Design review of the part built by this model. Coordinates are the model's own, in mm. A direction names the side the tool comes from. Coordinates: 2 decimals unless noted, no trailing zeros. Loops run counter-clockwise (first coordinate to the right, second up) from the corner with the lowest first, then second, coordinate; pieces in that order, holes last. Notation, with made-up numbers: (71.5, -27) -> (127.5, -27) arc R19 ccw to (127.5, -5) -> close; hole circle Ø8 at (43, 28.5). An arc over 180 degrees is marked (long way). One line per item, written item: value. Start each with the question number.
1. Add section A-A on x = 22. Write out the cut boundary in (y, z).
2. Draft analysis for pull direction Y (two halves, no side actions). For faces 4 (the cylindrical face through (31.1, -16.42, 11.15)), 5 (the cylindrical face through (26.06, -19.87, 12.63)), 6 (the flat face through (6, -23, 3)), state which applies: pulls with the +Y half, pulls with the -Y half, needs draft (parallel to the pull), parting line crosses it, or undercut.
3. Machinability: for faces 1 (the flat face through (31, -20.47, 12)), 2 (the cylindrical face through (-22.939, -10.265, 10.846)), 3 (the cylindrical face through (-13.08, -19.87, 12.63)), which of the approach directions +Z, -Z, +X, -X, +Y, -Y give a long, thin tool a straight path to every point of the face, cutting with its end or side? Answer none if there is none.
4. Insertion check: pin 1 (4 mm diameter, centred on x = 3.5, z = 7, fed in from -Y); pin 2 (3.5 mm diameter, centred on x = -18.5, z = 13, fed in from -Y); pin 3 (4 mm diameter, centred on x = -6, y = -21, fed in from +Z). Each pin has a flat end and moves straight along its axis. Give the tip position at first contact, or say it passes through.
5. Add section C-C on z = 16.75. Write out the cut boundary in (x, y), plus the area to 3 significant figures.
6. For probe 1 along Y at (x, z) = (-18.5, 17.75); probe 2 along X at (y, z) = (-13.25, 18.5); probe 3 along X at (y, z) = (-17, 16.75), list the stretches that pass through material, from the lowest coordinate up.
7. Add section D-D on y = -21.25. Write out the cut boundary in (x, z), plus the area to 3 significant figures.
8. Add section B-B on z = 2.25. Write out the cut boundary in (x, y).
```python
from build123d import *

# Parameters (mm, degrees)
SKETCH_1_W          = 60
SKETCH_1_H          = 20
SKETCH_1_R          = 1.5
EXTRUDE_2_DEPTH     = 3
EXTRUDE_3_DEPTH     = 19
SKETCH_3_R          = 1.8
CUT_EXTRUDE_1_DEPTH = 52.917907506
FILLET_1_R          = 2


with BuildPart() as part:
    # ｽｹｯﾁ1 → ﾎﾞｽ - 押し出し2 (new body)
    with BuildSketch(Plane.XY):
        with Locations((6.490384615, -19.663461538)):
            Rectangle(SKETCH_1_W, SKETCH_1_H)
        with Locations((30.990384615, -24.663461538)):
            Circle(SKETCH_1_R, mode=Mode.SUBTRACT)
        with Locations((-18.009615385, -24.663461538)):
            Circle(SKETCH_1_R, mode=Mode.SUBTRACT)
    extrude(amount=EXTRUDE_2_DEPTH)

    # ｽｹｯﾁ2 → ﾎﾞｽ - 押し出し3 (add)
    with BuildSketch(Plane.XY.offset(3)):
        Polygon((6.490384615, -16.663461538), (25.490384615, -16.663461538), (25.490384615, -20.47046126), (36.490384615, -20.47046126), (36.490384615, -9.663461538), (-23.509615385, -9.663461538), (-23.509615385, -20.47046126), (-12.509615385, -20.47046126), (-12.509615385, -16.663461538), align=None)
    extrude(amount=EXTRUDE_3_DEPTH)

    # ｽｹｯﾁ3 → ｶｯﾄ - 押し出し1 (cut, through all)
    with BuildSketch(Plane.XY.offset(22)):
        with Locations((31.490384615, -14.663461538)):
            Circle(SKETCH_3_R)
        with Locations((-18.509615385, -14.663461538)):
            Circle(SKETCH_3_R)
    extrude(amount=-CUT_EXTRUDE_1_DEPTH, mode=Mode.SUBTRACT)

    # ﾌｨﾚｯﾄ1
    fillet_1_edges = [part.edges().sort_by_distance(p)[0] for p in [
        (25.490384615, -20.47046126, 12.5),
        (36.490384615, -20.47046126, 12.5),
        (-23.509615385, -20.47046126, 12.5),
        (-12.509615385, -20.47046126, 12.5),
        (-23.509615385, -9.663461538, 11),
        (36.490384615, -9.663461538, 11),
        (36.490384615, -29.663461538, 1.5),
        (-23.509615385, -29.663461538, 1.5),
    ]]
    fillet(fillet_1_edges, radius=FILLET_1_R)


solid = part.part
```
Worked answers:
1. outline: (-29.66, 0) -> (-9.66, 0) -> (-9.66, 22) -> (-16.66, 22) -> (-16.66, 3) -> (-29.66, 3) -> close
2. face 4: undercut
2. face 5: pulls with the -Y half
2. face 6: needs draft
3. face 1: +Z, +X, -X, -Y
3. face 2: +Z, -Z, -X, +Y
3. face 3: +Z, -Y
4. pin 1: stops at y = -16.66
4. pin 2: stops at y = -20.47
4. pin 3: stops at z = 3
5. outline: (-23.51, -18.47) arc R2 ccw to (-21.51, -20.47) -> (-14.51, -20.47) arc R2 ccw to (-12.51, -18.47) -> (-12.51, -16.66) -> (25.49, -16.66) -> (25.49, -18.47) arc R2 ccw to (27.49, -20.47) -> (34.49, -20.47) arc R2 ccw to (36.49, -18.47) -> (36.49, -11.66) arc R2 ccw to (34.49, -9.66) -> (-21.51, -9.66) arc R2 ccw to (-23.51, -11.66) -> close; hole circle Ø3.6 at (-18.51, -14.66); hole circle Ø3.6 at (31.49, -14.66)
5. area: 478 mm²
6. probe 1: y = -20.47 to -16.46, -12.86 to -9.66
6. probe 2: x = -23.51 to -19.62, -17.4 to 30.38, 32.6 to 36.49
6. probe 3: x = -23.51 to -12.51, 25.49 to 36.49
7. outline: (-23.51, 0) -> (36.49, 0) -> (36.49, 3) -> (-23.51, 3) -> close
7. area: 180 mm²
8. outline: (-23.51, -27.66) arc R2 ccw to (-21.51, -29.66) -> (34.49, -29.66) arc R2 ccw to (36.49, -27.66) -> (36.49, -11.66) arc R2 ccw to (34.49, -9.66) -> (-21.51, -9.66) arc R2 ccw to (-23.51, -11.66) -> close; hole circle Ø3.6 at (-18.51, -14.66); hole circle Ø3 at (-18.01, -24.66); hole circle Ø3 at (30.99, -24.66); hole circle Ø3.6 at (31.49, -14.66)
